```python
from build123d import *

# Parameters (mm, degrees)
SKETCH_1_R      = 2.5
EXTRUDE_1_DEPTH = 5


with BuildPart() as part:
    # 草图1 → 凸台-拉伸1 (new body)
    with BuildSketch(Plane.XY.offset(5)):
        Polygon((15.930030419, -70.000000012), (15.930030419, -84.99999999), (90.930030476, -84.99999999), (105.930030424, -70.000000041), (105.930030424, 50.000000019), (90.930030476, 64.999999967), (15.930030419, 64.999999967), (15.930030419, 50.000000018), (-122.069969569, 50.000000018), (-122.069969569, 94.999999997), (-197.069969626, 94.999999997), (-212.069969578, 80.000000045), (-212.069969578, -100.000000045), (-197.069969626, -114.999999997), (-122.069969569, -114.999999997), (-122.069969569, -70.000000012), align=None)
        with Locations((-179.069969574, 80)):
            Circle(SKETCH_1_R, mode=Mode.SUBTRACT)
        with Locations(Location((-179.069969574, -100, 0), (0, 0, 180))):
            Circle(SKETCH_1_R, mode=Mode.SUBTRACT)
        with Locations(Location((72.930030422, -70.000000022, 0), (0, 0, 180))):
            Circle(SKETCH_1_R, mode=Mode.SUBTRACT)
        with Locations(Location((48.930030422, 50, 0), (0, 0, 180))):
            Circle(SKETCH_1_R, mode=Mode.SUBTRACT)
        with Locations(Location((-155.069969574, 80, 0), (0, 0, 180))):
            Circle(SKETCH_1_R, mode=Mode.SUBTRACT)
        with Locations((-155.069969574, -100)):
            Circle(SKETCH_1_R, mode=Mode.SUBTRACT)
        with Locations(Location((-65.069969575, -10, 0), (0, 0, 180))):
            Circle(SKETCH_1_R, mode=Mode.SUBTRACT)
        with Locations(Location((-41.069969575, -10.000000011, 0), (0, 0, 180))):
            Circle(SKETCH_1_R, mode=Mode.SUBTRACT)
        with Locations((72.930030422, 50)):
            Circle(SKETCH_1_R, mode=Mode.SUBTRACT)
        with Locations((48.930030422, -70.000000022)):
            Circle(SKETCH_1_R, mode=Mode.SUBTRACT)
    extrude(amount=-EXTRUDE_1_DEPTH)


solid = part.part
```
Source: CAD feature listing. Evaluate the final solid. Frame: model axes, mm. Coordinates: 2 decimals unless noted, no trailing zeros. Order: outer loops, then holes, each group sorted by start corner. A loop starts at its lowest first (then second) coordinate and runs counter-clockwise, first axis right, second up. Notation, with made-up numbers: (-5.75, 8.5) - (9.25, 8.5) arc R13 cw to (9.25, 23.5) - close; hole circle Ø4 at (41.25, 51.5). An arc over 180 degrees is marked (long way). One line per item, written item: value.
1) Cut plane C-C on x = -106. Output: boundary loops of the cut face in (y, z), plus the area to 3 significant figures.
Computed values:
outline: (-70, 0) - (50, 0) - (50, 5) - (-70, 5) - close
area: 600 mm^2
2) Ray query, line 1 (X direction, y = -10, z = 1.2); line 2 (X direction, y = 48.5, z = 3.4); line 3 (Y direction, x = -25, z = 1.9). Return the intervals inside material, ascending. Write a range as [from, to].
Computed values:
line 1: x = [-212.07, -67.57], [-62.57, -43.57], [-38.57, 105.93]
line 2: x = [-212.07, 46.93], [50.93, 70.93], [74.93, 105.93]
line 3: y = [-70, 50]
3) Contact query for flat-ended pins moving along their axis: pin 1 (6 mm diameter, centred on x = -179.07, y = -100, fed in from +Z); pin 2 (4 mm diameter, centred on x = 72.93, y = 50, fed in from +Z); pin 3 (2 mm diameter, centred on x = 23, z = 3.5, fed in from +Y); pin 4 (1.5 mm diameter, centred on y = -97.5, z = 3, fed in from +X). Output: stop coordinate, or through.
Computed values:
pin 1: stops at z = 5
pin 2: passes through
pin 3: stops at y = 65
pin 4: stops at x = -122.07
4) Cut plane B-B on y = -77. Output: boundary loops of the cut face in (x, z).
Computed values:
outline: (-212.07, 0) - (-122.07, 0) - (-122.07, 5) - (-212.07, 5) - close; (15.93, 0) - (98.93, 0) - (98.93, 5) - (15.93, 5) - close
5) Cut plane A-A on z = 2.7. State how many separate pieces and enclosed holes the cut face has, plus the area to 3 significant figures.
Computed values:
separate pieces: 1
enclosed holes: 10
area: 48,300 mm^2
6) Cut plane D-D on x = 86. Output: boundary loops of the cut face in (y, z).
Computed values:
outline: (-85, 0) - (65, 0) - (65, 5) - (-85, 5) - close
